For this review, take the finished solid that the model builds, in its own axes (mm). A direction names the side the tool comes from. Coordinates: 2 decimals unless noted, no trailing zeros. Loops run counter-clockwise (first coordinate to the right, second up) from the corner with the lowest first, then second, coordinate; pieces in that order, holes last. Notation, with made-up numbers: M 48.5,10 L 77.5,10 A18 ccw 77.5,21 Z; hole C -32.5,11.25 d11. An arc over 180 degrees is marked long. Put each result on its own line as item: value.
Autodesk Inventor part; units mm, degrees
ref_plane "YZ Plane" through (0, 0, 0) normal (1, 0, 0) x (0, 1, 0)
ref_plane "XZ Plane" through (0, 0, 0) normal (0, 1, 0) x (-1, 0, 0)
ref_plane "XY Plane" through (0, 0, 0) normal (0, 0, 1) x (1, 0, 0)
sketch "Sketch2" plane through (0, 0, 0) normal (0, 1, 0) x (-1, 0, 0)
  line L0 (12.7, 12.7) -> (-12.7, 12.7)
  line L1 (-12.7, 12.7) -> (-12.7, -12.7)
  line L2 (-12.7, -12.7) -> (12.7, -12.7)
  line L3 (12.7, -12.7) -> (12.7, 12.7)
  line L4 (12.7, 0) -> (-12.7, 0) construction
  line L5 (0, -12.7) -> (0, 12.7) construction
  point P0 (0, 0)
  point P1 (0, 0)
  dimension "d2" = 25.4
  dimension "d3" = 25.4
extrude "Base" add sketch "Sketch2" against normal blind 6.5
sketch "Sketch10" plane through (0, -6.5, 0) normal (0, -1, 0) x (1, 0, 0)
  line L0 (-12.7, -12.7) -> (12.7, -12.7)
  line L1 (12.7, -12.7) -> (12.7, 0)
  line L2 (12.7, 0) -> (6.35, 0)
  line L3 (6.35, 0) -> (6.35, -12.7)
  line L4 (6.35, -12.7) -> (12.7, -12.7)
  line L5 (0, -12.7) -> (6.35, -12.7)
  line L6 (6.35, -12.7) -> (6.35, -6.35)
  line L7 (6.35, -6.35) -> (0, -6.35)
  line L8 (0, -6.35) -> (0, -12.7)
  point P0 (0, 0)
  dimension "d44" = 6.35
  dimension "d45" = 12.7
  dimension "d46" = 6.35
  dimension "d47" = 6.35
extrude "Extrusion5" add sketch "Sketch10" along normal blind 6.35
sketch "Sketch11" plane through (0, 0, 0) normal (0, 1, 0) x (1, 0, 0)
  line L0 (12.7, -12.7) -> (-12.7, -12.7)
  line L1 (-12.7, -12.7) -> (-3.1541, -3.1541) construction
  line L2 (-12.7, -12.7) -> (0.8, -12.7) construction
  circle A0 centre (-3.1541, -3.1541) radius 5.5 construction
  point P0 (0, 0)
  dimension "d50" = 13.5
  dimension "d51" = 45
  dimension "d52" = 11
hole "Hole3" at (-3.1541, 0, 3.1541) direction (0, -1, 0) diameter 5.5 end through all countersink diameter 11 countersink angle 90
sketch "Sketch12" plane through (12.7, 0, -12.7) normal (0, 0, -1) x (-1, 0, 0)
  line L0 (12.7, -6.5) -> (12.7, -12.85)
  line L1 (0, -6.5) -> (25.4, -6.5) construction
  line L2 (12.7, -6.5) -> (0, -6.5)
  line L3 (0, -6.5) -> (0, -12.85) construction
  line L4 (0, -12.85) -> (5, -12.85) construction
  line L5 (5, -12.85) -> (5, -7.85) construction
  line L6 (5, -7.85) -> (0, -7.85) construction
  line L7 (0, -7.85) -> (0, -12.85) construction
  line L8 (5, -7.85) -> (0, -12.85) construction
  line L9 (5, -12.85) -> (0, -7.85) construction
  circle A0 centre (2.5, -10.35) radius 2.425
  point P0 (12.7, 0)
  dimension "d60" = 5
  dimension "d61" = 5
  dimension "d62" = 4.85
extrude "Extrusion6" add sketch "Sketch12" along normal blind 6.25
equation "\"d3\" = d2"
properties part number "Door pin right"
(1) Add section C-C (z = -10). Write out the cut boundary in (x, y), plus the area to 3 significant figures.
Determined:
outline: M -12.7,-6.5 L 0,-6.5 L 0,-12.85 L 12.7,-12.85 L 12.7,0 L -12.7,0 Z
area: 246 mm^2
(2) Add section A-A (x = 10.2). Write out the cut boundary in (y, z) (3 decimals).
Determined:
outline: M -12.85,-12.7 L -12.775,-12.7 L -12.775,-18.95 L -7.925,-18.95 L -7.925,-12.7 L 0,-12.7 L 0,12.7 L -6.5,12.7 L -6.5,0 L -12.85,0 Z
(3) Draft analysis for pull direction Z (two halves, no side actions). For faces 1 (the conical face through (-5.746, -2.578, 4.502)), 2 (the flat face through (10, -10, 0)), 3 (the cylindrical face through (8.896, -12.395, -15.781)), state which applies: +Z half, -Z half, draft (parallel to the pull), parting line (faces both ways), or undercut.
Determined:
face 1: undercut
face 2: +Z half
face 3: draft
(4) Add section D-D (y = -10.35). Write out the cut boundary in (x, z) (3 decimals), plus the area to 3 significant figures.
Determined:
outline: M 0,-12.7 L 7.775,-12.7 L 7.775,-18.95 L 12.625,-18.95 L 12.625,-12.7 L 12.7,-12.7 L 12.7,0 L 6.35,0 L 6.35,-6.35 L 0,-6.35 Z
area: 151 mm^2
(5) Tool access review of faces 4 (the flat face through (6.35, -10, -3)), 5 (the cylindrical face through (-0.47, -4.65, 2.56)), 6 (the flat face through (0, -10, -9)): name each direction out of +Z, -Z, +X, -X, +Y, -Y from which nothing blocks a thin tool from reaching the whole face with its end or side.
Determined:
face 4: +Z, -X, -Y
face 5: +Y, -Y
face 6: +Z, -Z, -X, -Y
(6) Wall thickness on line 1 along Y through (x, z) = (4, 4.5); line 2 along Z through (x, y) = (-8.5, -1.75); line 3 along X through (y, z) = (-11.25, -3.5): over which ranges is each line inside the solid? List them lowest first. Write a range as [from, to].
Determined:
line 1: y = [-6.5, 0]
line 2: z = [-12.7, 12.7]
line 3: x = [6.35, 12.7]
(7) Add section B-B (y = -1). Write out the cut boundary in (x, z), plus the area to 3 significant figures.
Determined:
outline: M -12.7,-12.7 L 12.7,-12.7 L 12.7,12.7 L -12.7,12.7 Z; hole C -3.15,3.15 d9
area: 582 mm^2
(8) For pin 1 (3 mm diameter, centred on x = 11, y = -10, fed in from +Z); pin 2 (5 mm diameter, centred on x = 2.5, y = -9.5, fed in from +Z); pin 3 (1.5 mm diameter, centred on x = -6.5, z = -2.5, fed in from -Y), all flat-tipped, find the tip position at first contact; note any pin that passes through.
Determined:
pin 1: stops at z = 0
pin 2: stops at z = -6.35
pin 3: stops at y = -6.5
